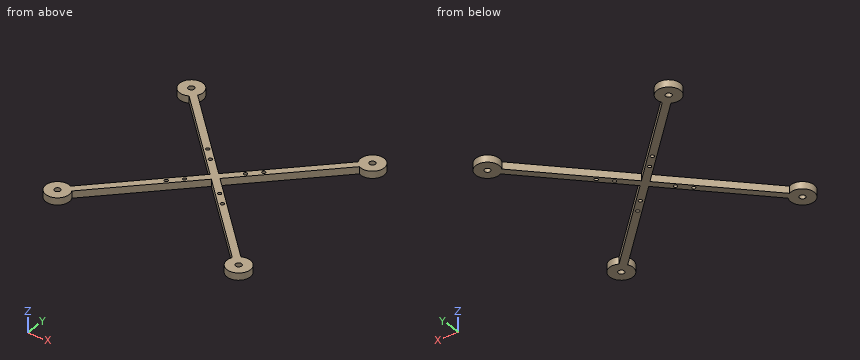
from build123d import *

# Parameters (mm, degrees)
SKETCH1_R           = 2.5
SKETCH1_R_2         = 1.5
BOSS_EXTRUDE1_DEPTH = 6


with BuildPart() as part:
    # Sketch1 → Boss-Extrude1 (new body)
    with BuildSketch(Plane.XY):
        with BuildLine():
            Line((-72.875951562, -68.633310875), (-4.242640687, 0))
            Line((-4.242640687, 0), (-72.875951562, 68.633310875))
            ThreePointArc((-72.875951562, 68.633310875), (-84.571067812, 84.571067812), (-68.633310875, 72.875951562))
            Line((-68.633310875, 72.875951562), (0, 4.242640687))
            Line((0, 4.242640687), (68.633310875, 72.875951562))
            ThreePointArc((68.633310875, 72.875951562), (84.571067812, 84.571067812), (72.875951562, 68.633310875))
            Line((72.875951562, 68.633310875), (4.242640687, 0))
            Line((4.242640687, 0), (72.875951562, -68.633310875))
            ThreePointArc((72.875951562, -68.633310875), (84.571067812, -84.571067812), (68.633310875, -72.875951562))
            Line((68.633310875, -72.875951562), (0, -4.242640687))
            Line((0, -4.242640687), (-68.633310875, -72.875951562))
            ThreePointArc((-68.633310875, -72.875951562), (-84.571067812, -84.571067812), (-72.875951562, -68.633310875))
        make_face()
        with Locations((-77.5, -77.5)):
            Circle(SKETCH1_R, mode=Mode.SUBTRACT)
        with Locations((-15, -15)):
            Circle(SKETCH1_R_2, mode=Mode.SUBTRACT)
        with Locations((-24, -24)):
            Circle(SKETCH1_R_2, mode=Mode.SUBTRACT)
        with Locations((-24, 24)):
            Circle(SKETCH1_R_2, mode=Mode.SUBTRACT)
        with Locations((-15, 15)):
            Circle(SKETCH1_R_2, mode=Mode.SUBTRACT)
        with Locations((-77.5, 77.5)):
            Circle(SKETCH1_R, mode=Mode.SUBTRACT)
        with Locations((24, 24)):
            Circle(SKETCH1_R_2, mode=Mode.SUBTRACT)
        with Locations((15, 15)):
            Circle(SKETCH1_R_2, mode=Mode.SUBTRACT)
        with Locations((77.5, 77.5)):
            Circle(SKETCH1_R, mode=Mode.SUBTRACT)
        with Locations((24, -24)):
            Circle(SKETCH1_R_2, mode=Mode.SUBTRACT)
        with Locations((15, -15)):
            Circle(SKETCH1_R_2, mode=Mode.SUBTRACT)
        with Locations((77.5, -77.5)):
            Circle(SKETCH1_R, mode=Mode.SUBTRACT)
    extrude(amount=BOSS_EXTRUDE1_DEPTH)


solid = part.part
Verification items for the finished model (mm, model axes). Give positions to 0.01 mm unless a question says otherwise; leave off trailing zeros. Loops run counter-clockwise (first coordinate to the right, second up) from the corner with the lowest first, then second, coordinate; pieces in that order, holes last.
1. Cross-section at C-C on x = -29. Record the cut outline in (y, z).
Derived:
outline: (-33.24, 0) - (-24.76, 0) - (-24.76, 6) - (-33.24, 6) - close; (24.76, 0) - (33.24, 0) - (33.24, 6) - (24.76, 6) - close
2. Go/stop test with flat-tipped pins: P1, Ø4, axis at x = 15, y = -15, coming from the +Z side; P2, Ø2.5, axis at x = 24, y = 24, coming from the -Z side; P3, Ø3, axis at y = -25, z = 1.5, coming from the +X side; P4, Ø1, axis at x = 49, z = 1.5, coming from the +Y side. Record where each tip stops, or that it passes through.
Derived:
P1: stops at z = 6
P2: passes through
P3: stops at x = 30.74
P4: stops at y = 53.74
3. Cross-section at A-A on y = -77.5. Record the cut outline in (x, z), and give its area (3 significant figures).
Derived:
outline: (-87.5, 0) - (-80, 0) - (-80, 6) - (-87.5, 6) - close; (-75, 0) - (-67.5, 0) - (-67.5, 6) - (-75, 6) - close; (67.5, 0) - (75, 0) - (75, 6) - (67.5, 6) - close; (80, 0) - (87.5, 0) - (87.5, 6) - (80, 6) - close
area: 180 mm2
4. Cross-section at D-D on y = -46.5. Record the cut outline in (x, z), and give its area (3 significant figures).
Derived:
outline: (-50.74, 0) - (-42.26, 0) - (-42.26, 6) - (-50.74, 6) - close; (42.26, 0) - (50.74, 0) - (50.74, 6) - (42.26, 6) - close
area: 102 mm2
5. Cross-section at B-B on z = 3.2. Count the separate pieces of the cut face and the enclosed holes in it, and give its area (3 significant figures).
Derived:
separate pieces: 1
enclosed holes: 12
area: 3,480 mm2
6. Material ranges on probe 1 along Y at (x, z) = (-77.5, 2.4); probe 2 along Y at (x, z) = (24, 3.5); probe 3 along X at (y, z) = (14.5, 2.2), recorded low to high.
Derived:
probe 1: y = -87.5 to -80, -75 to -67.5, 67.5 to 75, 80 to 87.5
probe 2: y = -28.24 to -25.5, -22.5 to -19.76, 19.76 to 22.5, 25.5 to 28.24
probe 3: x = -18.74 to -16.41, -13.59 to -10.26, 10.26 to 13.59, 16.41 to 18.74
